Design review of the part built by this model. Coordinates are the model's own, in mm. A direction names the side the tool comes from. Round coordinates to 2 decimals unless told otherwise and drop trailing zeros. Loops run counter-clockwise (first coordinate to the right, second up) from the corner with the lowest first, then second, coordinate; pieces in that order, holes last. Notation, with made-up numbers: (82.25, 36.25) -> (117.25, 36.25) arc R24 ccw to (117.25, 54.25) -> close; hole circle Ø10 at (-8.75, -23). An arc over 180 degrees is marked (long way). Answer as CSV lines item,"result". Start each with the question number.
Autodesk Inventor part; units mm, degrees
ref_plane "YZ Plane" through (0, 0, 0) normal (1, 0, 0) x (0, 1, 0)
ref_plane "XZ Plane" through (0, 0, 0) normal (0, 1, 0) x (-1, 0, 0)
ref_plane "XY Plane" through (0, 0, 0) normal (0, 0, 1) x (1, 0, 0)
sketch "スケッチ1" plane through (0, 0, 0) normal (0, 0, 1) x (1, 0, 0)
  line L0 (0, 0) -> (6, 0)
  line L1 (6, 0) -> (6, 1.5)
  line L2 (6, 1.5) -> (0, 1.5)
  line L3 (0, 1.5) -> (0, 0)
  line L4 (0, 0) -> (0, 2.75)
  line L5 (0, 0) -> (-2, 0)
  line L6 (-2, 0) -> (0, 0)
  line L7 (-2, 0) -> (-2, 1.15)
  arc A0 (0, 2.75) -> (-2, 1.15) centre (-0.0403, 0.7504) ccw
  dimension "d0" = 1.5
  dimension "d1" = 6
  dimension "d3" = 2
  dimension "d4" = 2.75
  dimension "d5" = 1.15
  dimension "d6" = 2
revolve "回転1" add sketch "スケッチ1" angle 360 about axis through (-2, 0, 0) along (1, 0, 0)
thread "ねじ1"
sketch "スケッチ2" plane through (-2, 0, 0) normal (-1, 0, 0) x (0, 0, 1)
  circle A0 centre (0, 0) radius 1.15
  line L0 (-0.575, 0.9959) -> (0.575, 0.9959)
  line L1 (0.575, 0.9959) -> (1.15, 0)
  line L2 (1.15, 0) -> (0.575, -0.9959)
  line L3 (0.575, -0.9959) -> (-0.575, -0.9959)
  line L4 (-0.575, -0.9959) -> (-1.15, 0)
  line L5 (-1.15, 0) -> (-0.575, 0.9959)
  dimension "d10" = 1.15
  dimension "d11" = 1.9919
extrude "押し出し1" cut sketch "スケッチ2" against normal blind 1.4 contours L2 L3 L4 L5 L0 L1
fillet "フィレット1" radius 0.2 6 edges at (-0.6, 0.9959, 0) (-0.6, 0.498, 0.8625) (-0.6, 0.498, -0.8625) (-0.6, -0.498, -0.8625) (-0.6, -0.9959, 0) (-0.6, -0.498, 0.8625)
fillet "フィレット2" radius 0.1 1 edges at (0, -1.5, 0)
fillet "フィレット3" radius 0.1 1 edges at (6, -1.5, 0)
properties part number "ネジボタンM3L6" material "鋼"
Q1. Add section A-A, the plane x = 4.75. Give the boundary of the cut face in (y, z), and give its area (3 significant figures).
Q2. To check wall thickness, follow probe 1 along Z at (x, y) = (-0.75, 0.5); probe 2 along X at (y, z) = (-0.05, 0.9); probe 3 along X at (y, z) = (0.15, 1.6). State the ranges of each line that lie inside material, in increasing order. Write a range as from..to.
Q3. For pin 1 Ø0.6 at (x, z) = (-1.5, 0) entering from +Y; pin 2 Ø1.5 at (x, z) = (-1, 2) entering from -Y; pin 3 Ø0.6 at (x, z) = (-1.5, 0) entering from -Y, all flat-tipped, find the tip position at first contact; note any pin that passes through.
Q4. Machinability: for faces 4 (the flat face through (-1.408, 0.491, -0.867)), 5 (the flat face through (0, 2, 0)), which of the approach directions +Z, -Z, +X, -X, +Y, -Y give a long, thin tool a straight path to every point of the face, cutting with its end or side? Answer none if there is none.
Q5. Mouldability with a two-part tool opening along Y and no side actions: class faces 1 (the cylindrical face through (2.96, -1.5, -0.07)), 2 (the flat face through (-1.41, -0.5, -0.86)), 3 (the flat face through (6, 0, 0)) as pulls with the +Y half, pulls with the -Y half, needs draft (parallel to the pull), parting line crosses it, or undercut.
Worked answers:
1,outline,"circle Ø3 at (0, 0)"
1,area,"7.07 mm^2"
2,probe 1,"z = -2.57..-0.85, 0.85..2.57"
2,probe 2,"x = -0.6..6"
2,probe 3,"x = -1.85..0"
3,pin 1,"stops at y = 2.38"
3,pin 2,"stops at y = -2.3"
3,pin 3,"stops at y = -2.38"
4,face 4,"-X"
4,face 5,"+X"
5,face 1,"parting line crosses it"
5,face 2,"undercut"
5,face 3,"needs draft"
